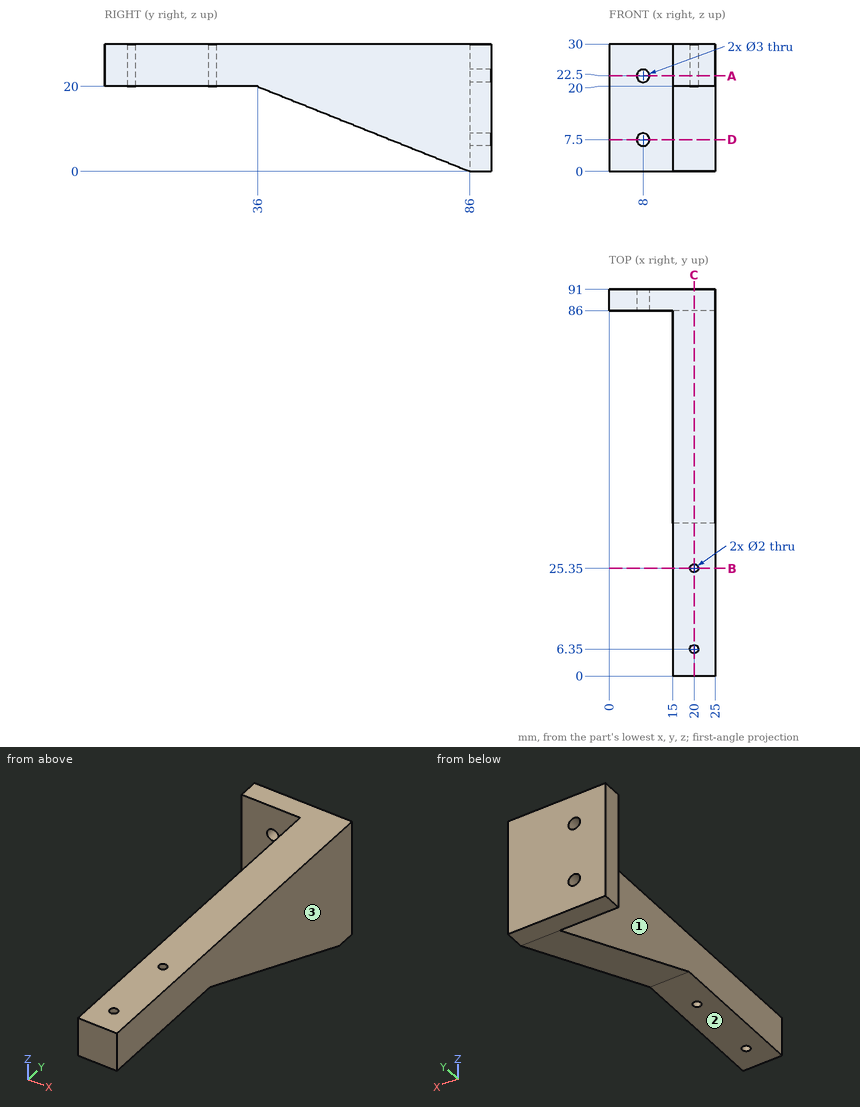
Geometry: see drawing. Coordinates: mm, zero at the bounding-box minimum. A direction names the side the tool comes from. Give positions to 0.01 mm unless a question says otherwise; leave off trailing zeros. Order: outer loops, then holes, each group sorted by start corner. A loop starts at its lowest first (then second) coordinate and runs counter-clockwise, first axis right, second up. Notation, with made-up numbers: (75.25, 39) -> (134.25, 39) arc R20 ccw to (134.25, 66) -> close; hole circle Ø3 at (81, 28.5). An arc over 180 degrees is marked (long way). Write each question's results on one line, items separated by ' | '. Start each with the question number.
1) Section B-B (y = 25.35). Return loops of the section in (x, z).
2) First-contact query: pin 1 (12 mm diameter, centred on x = 21.5, y = 41, fed in from -Z); pin 2 (5 mm diameter, centred on x = 8, z = 22.5, fed in from -Y); pin 3 (2.5 mm diameter, centred on x = 20, y = 25.35, fed in from -Z). Flat tips, straight axial feed; report the tip coordinate or a pass-through.
3) Line query: line 1 (Z direction, x = 8, y = 88.2); line 2 (X direction, y = 25.35, z = 25.75); line 3 (Z direction, x = 18.75, y = 23). Output: solid intervals per line, ascending. Write a range as from..to.
4) Section C-C (x = 20). Return loops of the section in (y, z).
5) Section D-D (z = 7.5). Return loops of the section in (x, y).
6) Section A-A (z = 22.5). Return loops of the section in (x, y), then the cut area to 3 significant figures.
7) Set-up query: the marked faces 1, 2 and 3. Return all of +Z, -Z, +X, -X, +Y, -Y with unobstructed straight access to the full face (end or side cutting, diameter ignored); none if empty.
Calculated:
1) outline: (15, 20) -> (19, 20) -> (19, 30) -> (15, 30) -> close; (21, 20) -> (25, 20) -> (25, 30) -> (21, 30) -> close
2) pin 1: z = 15.6 | pin 2: y = 86 | pin 3: z = 20
3) line 1: 0..6, 9..21, 24..30 | line 2: 15..19, 21..25 | line 3: 20..30
4) outline: (0, 20) -> (5.35, 20) -> (5.35, 30) -> (0, 30) -> close; (7.35, 20) -> (24.35, 20) -> (24.35, 30) -> (7.35, 30) -> close; (26.35, 20) -> (36, 20) -> (86, 0) -> (91, 0) -> (91, 30) -> (26.35, 30) -> close
5) outline: (0, 86) -> (6.5, 86) -> (6.5, 91) -> (0, 91) -> close; (9.5, 86) -> (15, 86) -> (15, 67.25) -> (25, 67.25) -> (25, 91) -> (9.5, 91) -> close
6) outline: (0, 86) -> (6.5, 86) -> (6.5, 91) -> (0, 91) -> close; (9.5, 86) -> (15, 86) -> (15, 0) -> (25, 0) -> (25, 91) -> (9.5, 91) -> close; hole circle Ø2 at (20, 6.35); hole circle Ø2 at (20, 25.35) | area: 964 mm2
7) face 1: +Z, -Z, -X, -Y | face 2: -Z, +X, -X, -Y | face 3: +Z, -Z, +X, +Y, -Y
